```python
from build123d import *

# Parameters (mm, degrees)
F0_W     = 88
F0_H     = 90
F0_R     = 4.5
F0_R_2   = 4
F0_R_3   = 4.6
F0_R_4   = 4.7
F0_R_5   = 4.1
F0_R_6   = 4.2
F0_R_7   = 3.5
F0_R_8   = 3.6
F0_R_9   = 3.7
F0_R_10  = 4.8
F0_R_11  = 4.3
F0_R_12  = 4.9
F0_R_13  = 4.4
F0_R_14  = 3.8
F0_R_15  = 3.9
F0_R_16  = 3
F0_R_17  = 2.5
F0_R_18  = 3.05
F0_R_19  = 2.55
F0_R_20  = 2
F0_R_21  = 2.05
F0_R_22  = 3.1
F0_R_23  = 3.15
F0_R_24  = 2.6
F0_R_25  = 2.65
F0_R_26  = 3.2
F0_R_27  = 2.7
F0_R_28  = 2.1
F0_R_29  = 2.15
F0_R_30  = 2.2
F0_R_31  = 1.5
F0_R_32  = 1.55
F0_R_33  = 1
F0_R_34  = 0.5
F0_R_35  = 1.05
F0_R_36  = 0.55
F0_R_37  = 1.6
F0_R_38  = 1.65
F0_R_39  = 1.7
F0_R_40  = 1.1
F0_R_41  = 1.15
F0_R_42  = 0.6
F0_R_43  = 0.65
F0_R_44  = 1.2
F0_R_45  = 0.7
F0_R_46  = 3.25
F0_R_47  = 2.75
F0_R_48  = 3.3
F0_R_49  = 3.35
F0_R_50  = 2.8
F0_R_51  = 2.85
F0_R_52  = 2.25
F0_R_53  = 2.3
F0_R_54  = 2.35
F0_R_55  = 3.4
F0_R_56  = 2.9
F0_R_57  = 3.45
F0_R_58  = 2.95
F0_R_59  = 2.4
F0_R_60  = 2.45
F0_R_61  = 1.75
F0_R_62  = 1.8
F0_R_63  = 1.85
F0_R_64  = 1.25
F0_R_65  = 0.75
F0_R_66  = 1.3
F0_R_67  = 1.35
F0_R_68  = 0.8
F0_R_69  = 0.85
F0_R_70  = 1.9
F0_R_71  = 1.95
F0_R_72  = 1.4
F0_R_73  = 0.9
F0_R_74  = 1.45
F0_R_75  = 0.95
F1_DEPTH = 10


with BuildPart() as f1:
    # F0 (on Top) → F1 (new body)
    with BuildSketch(Plane.XY):
        Rectangle(F0_W, F0_H)
        with Locations((-36, -36)):
            Circle(F0_R, mode=Mode.SUBTRACT)
        with Locations((-36, -23)):
            Circle(F0_R_2, mode=Mode.SUBTRACT)
        with Locations((-20, -36)):
            Circle(F0_R_3, mode=Mode.SUBTRACT)
        with Locations((-4, -36)):
            Circle(F0_R_4, mode=Mode.SUBTRACT)
        with Locations((-20, -23)):
            Circle(F0_R_5, mode=Mode.SUBTRACT)
        with Locations((-4, -23)):
            Circle(F0_R_6, mode=Mode.SUBTRACT)
        with Locations((-36, -11)):
            Circle(F0_R_7, mode=Mode.SUBTRACT)
        with Locations((-20, -11)):
            Circle(F0_R_8, mode=Mode.SUBTRACT)
        with Locations((-4, -11)):
            Circle(F0_R_9, mode=Mode.SUBTRACT)
        with Locations((12, -36)):
            Circle(F0_R_10, mode=Mode.SUBTRACT)
        with Locations((12, -23)):
            Circle(F0_R_11, mode=Mode.SUBTRACT)
        with Locations((28, -36)):
            Circle(F0_R_12, mode=Mode.SUBTRACT)
        with Locations((28, -23)):
            Circle(F0_R_13, mode=Mode.SUBTRACT)
        with Locations((12, -11)):
            Circle(F0_R_14, mode=Mode.SUBTRACT)
        with Locations((28, -11)):
            Circle(F0_R_15, mode=Mode.SUBTRACT)
        with Locations((-36, 0)):
            Circle(F0_R_16, mode=Mode.SUBTRACT)
        with Locations((-36, 10)):
            Circle(F0_R_17, mode=Mode.SUBTRACT)
        with Locations((-28, 0)):
            Circle(F0_R_18, mode=Mode.SUBTRACT)
        with Locations((-28, 10)):
            Circle(F0_R_19, mode=Mode.SUBTRACT)
        with Locations((-36, 19)):
            Circle(F0_R_20, mode=Mode.SUBTRACT)
        with Locations((-28, 19)):
            Circle(F0_R_21, mode=Mode.SUBTRACT)
        with Locations((-20, 0)):
            Circle(F0_R_22, mode=Mode.SUBTRACT)
        with Locations((-12, 0)):
            Circle(F0_R_23, mode=Mode.SUBTRACT)
        with Locations((-20, 10)):
            Circle(F0_R_24, mode=Mode.SUBTRACT)
        with Locations((-12, 10)):
            Circle(F0_R_25, mode=Mode.SUBTRACT)
        with Locations((-4, 0)):
            Circle(F0_R_26, mode=Mode.SUBTRACT)
        with Locations((-4, 10)):
            Circle(F0_R_27, mode=Mode.SUBTRACT)
        with Locations((-20, 19)):
            Circle(F0_R_28, mode=Mode.SUBTRACT)
        with Locations((-12, 19)):
            Circle(F0_R_29, mode=Mode.SUBTRACT)
        with Locations((-4, 19)):
            Circle(F0_R_30, mode=Mode.SUBTRACT)
        with Locations((-36, 27)):
            Circle(F0_R_31, mode=Mode.SUBTRACT)
        with Locations((-28, 27)):
            Circle(F0_R_32, mode=Mode.SUBTRACT)
        with Locations((-36, 34)):
            Circle(F0_R_33, mode=Mode.SUBTRACT)
        with Locations((-36, 40)):
            Circle(F0_R_34, mode=Mode.SUBTRACT)
        with Locations((-28, 34)):
            Circle(F0_R_35, mode=Mode.SUBTRACT)
        with Locations((-28, 40)):
            Circle(F0_R_36, mode=Mode.SUBTRACT)
        with Locations((-20, 27)):
            Circle(F0_R_37, mode=Mode.SUBTRACT)
        with Locations((-12, 27)):
            Circle(F0_R_38, mode=Mode.SUBTRACT)
        with Locations((-4, 27)):
            Circle(F0_R_39, mode=Mode.SUBTRACT)
        with Locations((-20, 34)):
            Circle(F0_R_40, mode=Mode.SUBTRACT)
        with Locations((-12, 34)):
            Circle(F0_R_41, mode=Mode.SUBTRACT)
        with Locations((-20, 40)):
            Circle(F0_R_42, mode=Mode.SUBTRACT)
        with Locations((-12, 40)):
            Circle(F0_R_43, mode=Mode.SUBTRACT)
        with Locations((-4, 34)):
            Circle(F0_R_44, mode=Mode.SUBTRACT)
        with Locations((-4, 40)):
            Circle(F0_R_45, mode=Mode.SUBTRACT)
        with Locations((4, 0)):
            Circle(F0_R_46, mode=Mode.SUBTRACT)
        with Locations((4, 10)):
            Circle(F0_R_47, mode=Mode.SUBTRACT)
        with Locations((12, 0)):
            Circle(F0_R_48, mode=Mode.SUBTRACT)
        with Locations((20, 0)):
            Circle(F0_R_49, mode=Mode.SUBTRACT)
        with Locations((12, 10)):
            Circle(F0_R_50, mode=Mode.SUBTRACT)
        with Locations((20, 10)):
            Circle(F0_R_51, mode=Mode.SUBTRACT)
        with Locations((4, 19)):
            Circle(F0_R_52, mode=Mode.SUBTRACT)
        with Locations((12, 19)):
            Circle(F0_R_53, mode=Mode.SUBTRACT)
        with Locations((20, 19)):
            Circle(F0_R_54, mode=Mode.SUBTRACT)
        with Locations((28, 0)):
            Circle(F0_R_55, mode=Mode.SUBTRACT)
        with Locations((28, 10)):
            Circle(F0_R_56, mode=Mode.SUBTRACT)
        with Locations((36, 0)):
            Circle(F0_R_57, mode=Mode.SUBTRACT)
        with Locations((36, 10)):
            Circle(F0_R_58, mode=Mode.SUBTRACT)
        with Locations((28, 19)):
            Circle(F0_R_59, mode=Mode.SUBTRACT)
        with Locations((36, 19)):
            Circle(F0_R_60, mode=Mode.SUBTRACT)
        with Locations((4, 27)):
            Circle(F0_R_61, mode=Mode.SUBTRACT)
        with Locations((12, 27)):
            Circle(F0_R_62, mode=Mode.SUBTRACT)
        with Locations((20, 27)):
            Circle(F0_R_63, mode=Mode.SUBTRACT)
        with Locations((4, 34)):
            Circle(F0_R_64, mode=Mode.SUBTRACT)
        with Locations((4, 40)):
            Circle(F0_R_65, mode=Mode.SUBTRACT)
        with Locations((12, 34)):
            Circle(F0_R_66, mode=Mode.SUBTRACT)
        with Locations((20, 34)):
            Circle(F0_R_67, mode=Mode.SUBTRACT)
        with Locations((12, 40)):
            Circle(F0_R_68, mode=Mode.SUBTRACT)
        with Locations((20, 40)):
            Circle(F0_R_69, mode=Mode.SUBTRACT)
        with Locations((28, 27)):
            Circle(F0_R_70, mode=Mode.SUBTRACT)
        with Locations((36, 27)):
            Circle(F0_R_71, mode=Mode.SUBTRACT)
        with Locations((28, 34)):
            Circle(F0_R_72, mode=Mode.SUBTRACT)
        with Locations((28, 40)):
            Circle(F0_R_73, mode=Mode.SUBTRACT)
        with Locations((36, 34)):
            Circle(F0_R_74, mode=Mode.SUBTRACT)
        with Locations((36, 40)):
            Circle(F0_R_75, mode=Mode.SUBTRACT)
    extrude(amount=F1_DEPTH)


solid = f1.part
```
Geometry: final body of the model. Coordinates: model frame, mm. Round coordinates to 2 decimals unless told otherwise and drop trailing zeros. Order: outer loops, then holes, each group sorted by start corner. A loop starts at its lowest first (then second) coordinate and runs counter-clockwise, first axis right, second up. Notation, with made-up numbers: (34, -8.75) -> (75, -8.75) arc R38 ccw to (75, 30.25) -> close; hole circle Ø6 at (42, -21). An arc over 180 degrees is marked (long way). Use one line per item in the form item = value.
(1) Section B-B on z = 7.25. Count the separate pieces of the cut face and the enclosed holes in it, and give its area (3 significant figures).
Results list:
separate_pieces = 1
enclosed_holes = 75
area = 6,200 mm^2
(2) Draft query along X for faces 1 (the face through (44, -1, 5)), 2 (the face through (-27.17, 28.31, 4.93)), 3 (the face through (-1, 45, 5)). Return one class per face: pulls with the +X half, pulls with the -X half, needs draft (parallel to the pull), parting line crosses it, or undercut.
Results list:
face_1 = pulls with the +X half
face_2 = undercut
face_3 = needs draft
(3) Ray query, probe 1 along Y at (x, z) = (38, 2.25); probe 2 along Y at (x, z) = (24, 0.5); probe 3 along X at (y, z) = (-38, 3). Return the intervals inside material, ascending. Write a range as [from, to].
Results list:
probe_1 = [-45, -2.81], [2.81, 7.83], [12.17, 17.58], [20.42, 45]
probe_2 = [-45, -38.83], [-33.17, -24.83], [-21.17, 45]
probe_3 = [-44, -40.03], [-31.97, -24.14], [-15.86, -8.25], [0.25, 7.64], [16.36, 23.53], [32.47, 44]
(4) Section C-C on y = -11. Return loops of the section in (x, z), and give its area (3 significant figures).
Results list:
outline = (-44, 0) -> (-39.5, 0) -> (-39.5, 10) -> (-44, 10) -> close; (-32.5, 0) -> (-23.6, 0) -> (-23.6, 10) -> (-32.5, 10) -> close; (-16.4, 0) -> (-7.7, 0) -> (-7.7, 10) -> (-16.4, 10) -> close; (-0.3, 0) -> (8.2, 0) -> (8.2, 10) -> (-0.3, 10) -> close; (15.8, 0) -> (24.1, 0) -> (24.1, 10) -> (15.8, 10) -> close; (31.9, 0) -> (44, 0) -> (44, 10) -> (31.9, 10) -> close
area = 510 mm^2
(5) Section A-A on y = -23. Return loops of the section in (x, z).
Results list:
outline = (-44, 0) -> (-40, 0) -> (-40, 10) -> (-44, 10) -> close; (-32, 0) -> (-24.1, 0) -> (-24.1, 10) -> (-32, 10) -> close; (-15.9, 0) -> (-8.2, 0) -> (-8.2, 10) -> (-15.9, 10) -> close; (0.2, 0) -> (7.7, 0) -> (7.7, 10) -> (0.2, 10) -> close; (16.3, 0) -> (23.6, 0) -> (23.6, 10) -> (16.3, 10) -> close; (32.4, 0) -> (44, 0) -> (44, 10) -> (32.4, 10) -> close
